Verification items for the finished model (mm, model axes). A direction names the side the tool comes from. Coordinates: 2 decimals unless noted, no trailing zeros. Order: outer loops, then holes, each group sorted by start corner. A loop starts at its lowest first (then second) coordinate and runs counter-clockwise, first axis right, second up. Notation, with made-up numbers: M 2,80 L 21,80 A28 cw 21,107 Z; hole C -21,89.25 d3. An arc over 180 degrees is marked long. Return JSON: item names as keys, results as strings. Group by question number.
1. Section check A-A, the plane y = 35. Record the cut outline in (x, z) (3 decimals).
2. Gauge pin test, flat ends, axial feed: pin 1 (0.7 mm diameter, centred on y = -21, z = 4, fed in from -X); pin 2 (6 mm diameter, centred on x = -5.5, z = 2, fed in from +Y); pin 3 (8 mm diameter, centred on x = 0, y = -35, fed in from -Z); pin 4 (1 mm diameter, centred on x = -1, y = -40, fed in from +Z). Record the tip position at first contact, or that the pin passes through.
3. Section check C-C, the plane y = -22. Record the cut outline in (x, z) (1 decimal).
4. Mould release check, pull along Y, two halves, no side actions. Record for faces 1 (the flat face through (4.1, -46, 4)), 2 (the flat face through (8, -10, 3)): +Y half, -Y half, draft (parallel to the pull), parting line (faces both ways), or undercut.
5. Set-up check for faces 3 (the flat face through (4.1, 19, 4)), 4 (the flat face through (8, 0, -1)), 5 (the cylindrical face through (7.5, 35.1, 3.9)), 6 (the flat face through (-6, -45, 2.8)): record each of +Z, -Z, +X, -X, +Y, -Y from which the full face is reachable in a straight line by a thin tool's end or side.
6. Material ranges on line 1 along Y through (x, z) = (0, -3.05); line 2 along Z through (x, y) = (7.5, 17); line 3 along X through (y, z) = (35, -2.95), recorded low to high.
7. Section check B-B, the plane x = 0. Record the cut outline in (y, z), plus the area to 3 significant figures.
Autodesk Inventor part; units mm, degrees
ref_plane "side_1_XY" through (0, 0, -5) normal (0, 0, -1) x (-1, 0, 0)
ref_plane "side_1_YZ" through (0, 0, -5) normal (-1, 0, 0) x (0, 1, 0)
ref_plane "side_1_ZX" through (0, 0, -5) normal (0, 1, 0) x (0, 0, -1)
sketch "Skizze_1" plane through (0, 0, 0) normal (0, 1, 0) x (-1, 0, 0)
  arc A0 (10, 3.4) -> (8.4, 5) centre (8.4, 3.4) ccw
  line L0 (8.4, 5) -> (4.1, 5)
  line L1 (4.1, 5) -> (4.1, 2.8)
  line L2 (4.1, 2.8) -> (7.3, 2.8)
  arc A1 (7.795, 1.605) -> (7.3, 2.8) centre (7.3, 2.1) ccw
  line L3 (7.795, 1.605) -> (5.2757, -0.9142)
  arc A2 (3.8615, -1.5) -> (5.2757, -0.9142) centre (3.8615, 0.5) ccw
  line L4 (3.8615, -1.5) -> (-3.8615, -1.5)
  arc A3 (-5.2757, -0.9142) -> (-3.8615, -1.5) centre (-3.8615, 0.5) ccw
  line L5 (-5.2757, -0.9142) -> (-7.795, 1.605)
  arc A4 (-7.3, 2.8) -> (-7.795, 1.605) centre (-7.3, 2.1) ccw
  line L6 (-7.3, 2.8) -> (-4.1, 2.8)
  line L7 (-4.1, 2.8) -> (-4.1, 5)
  line L8 (-4.1, 5) -> (-8.4, 5)
  arc A5 (-8.4, 5) -> (-10, 3.4) centre (-8.4, 3.4) ccw
  line L9 (-10, 3.4) -> (-10, -3.4)
  arc A6 (-10, -3.4) -> (-8.4, -5) centre (-8.4, -3.4) ccw
  line L10 (-8.4, -5) -> (8.4, -5)
  arc A7 (8.4, -5) -> (10, -3.4) centre (8.4, -3.4) ccw
  line L11 (10, -3.4) -> (10, 3.4)
extrude "Extrusion1" add sketch "Skizze_1" along normal mid plane 100
sketch "Skizze_2" plane through (0, 0, 0) normal (1, 0, 0) x (0, 1, 0)
  line L0 (10, 9) -> (-10, 9)
  line L1 (-10, 9) -> (-10, -1)
  line L2 (-10, -1) -> (10, -1)
  line L3 (10, -1) -> (10, 9)
extrude "Extrusion2" cut sketch "Skizze_2" along normal blind 15
sketch "Skizze_3_ALT_Drilling_1" plane through (0, 0, 0) normal (0, 0, 1) x (1, 0, 0)
  circle A0 centre (0, -35) radius 4.5
extrude "Extrusion3" cut sketch "Skizze_3_ALT_Drilling_1" against normal blind 10
sketch "Skizze_4_ALT_Drilling_2" plane through (0, 0, 0) normal (0, 0, 1) x (1, 0, 0)
  circle A0 centre (0, 35) radius 4.5
extrude "Extrusion4" cut sketch "Skizze_4_ALT_Drilling_2" against normal blind 10
sketch "Skizze_5_ALT_Drilling_3" plane through (0, 0, -1.5) normal (0, 0, 1) x (1, 0, 0)
  circle A0 centre (0, 35) radius 7.5
extrude "Extrusion5" cut sketch "Skizze_5_ALT_Drilling_3" along normal blind 10
sketch "Skizze_6_ALT_Drilling_4" plane through (0, 0, -1.5) normal (0, 0, 1) x (1, 0, 0)
  circle A0 centre (0, -35) radius 7.5
extrude "Extrusion6" cut sketch "Skizze_6_ALT_Drilling_4" along normal blind 10
ref_plane "side_1_XY" through (0, 0, -5) normal (0, 0, -1) x (-1, 0, 0)
ref_plane "side_1_YZ" through (0, 0, -5) normal (-1, 0, 0) x (0, 1, 0)
ref_plane "side_1_ZX" through (0, 0, -5) normal (0, 1, 0) x (0, 0, -1)
ref_plane "side_6a_XY" through (0, 35, 5) normal (0, 0, 1) x (1, 0, 0)
ref_plane "side_6a_YZ" through (0, 35, 5) normal (1, 0, 0) x (0, 1, 0)
ref_plane "side_6a_ZX" through (0, 35, 5) normal (0, 1, 0) x (0, 0, 1)
ref_plane "side_6b_XY" through (0, -35, 5) normal (0, 0, 1) x (1, 0, 0)
ref_plane "side_6b_YZ" through (0, -35, 5) normal (1, 0, 0) x (0, 1, 0)
ref_plane "side_6b_ZX" through (0, -35, 5) normal (0, 1, 0) x (0, 0, 1)
properties part number "MayTec 1.68.201050_Hanging bracket"
Answers follow:
{
 "1": {"outline": "M -10,-3.4 A1.6 ccw -8.4,-5 L -4.5,-5 L -4.5,-1.5 L -7.5,-1.5 L -7.5,1.31 L -7.795,1.605 A0.7 cw -7.5,2.771 L -7.5,5 L -8.4,5 A1.6 ccw -10,3.4 Z; M 4.5,-5 L 8.4,-5 A1.6 ccw 10,-3.4 L 10,3.4 A1.6 ccw 8.4,5 L 7.5,5 L 7.5,2.771 A0.7 cw 7.795,1.605 L 7.5,1.31 L 7.5,-1.5 L 4.5,-1.5 Z"},
 "2": {"pin 1": "x = -9.98", "pin 2": "y = 50", "pin 3": "through", "pin 4": "z = -1.5"},
 "3": {"outline": "M -10,-3.4 A1.6 ccw -8.4,-5 L 8.4,-5 A1.6 ccw 10,-3.4 L 10,3.4 A1.6 ccw 8.4,5 L 4.1,5 L 4.1,2.8 L 7.3,2.8 A0.7 cw 7.8,1.6 L 5.3,-0.9 A2 cw 3.9,-1.5 L -3.9,-1.5 A2 cw -5.3,-0.9 L -7.8,1.6 A0.7 cw -7.3,2.8 L -4.1,2.8 L -4.1,5 L -8.4,5 A1.6 ccw -10,3.4 Z"},
 "4": {"face 1": "draft", "face 2": "undercut"},
 "5": {"face 3": "+Z, +Y, -Y", "face 4": "+Z, +X", "face 5": "+Z", "face 6": "+Y, -Y"},
 "6": {"line 1": "-50 to -39.5, -30.5 to 30.5, 39.5 to 50", "line 2": "-5 to 1.31, 2.77 to 5", "line 3": "-10 to -4.5, 4.5 to 10"},
 "7": {"outline": "M -50,-5 L -39.5,-5 L -39.5,-1.5 L -50,-1.5 Z; M -30.5,-5 L 30.5,-5 L 30.5,-1.5 L -30.5,-1.5 Z; M 39.5,-5 L 50,-5 L 50,-1.5 L 39.5,-1.5 Z", "area": "287 mm^2"}
}
